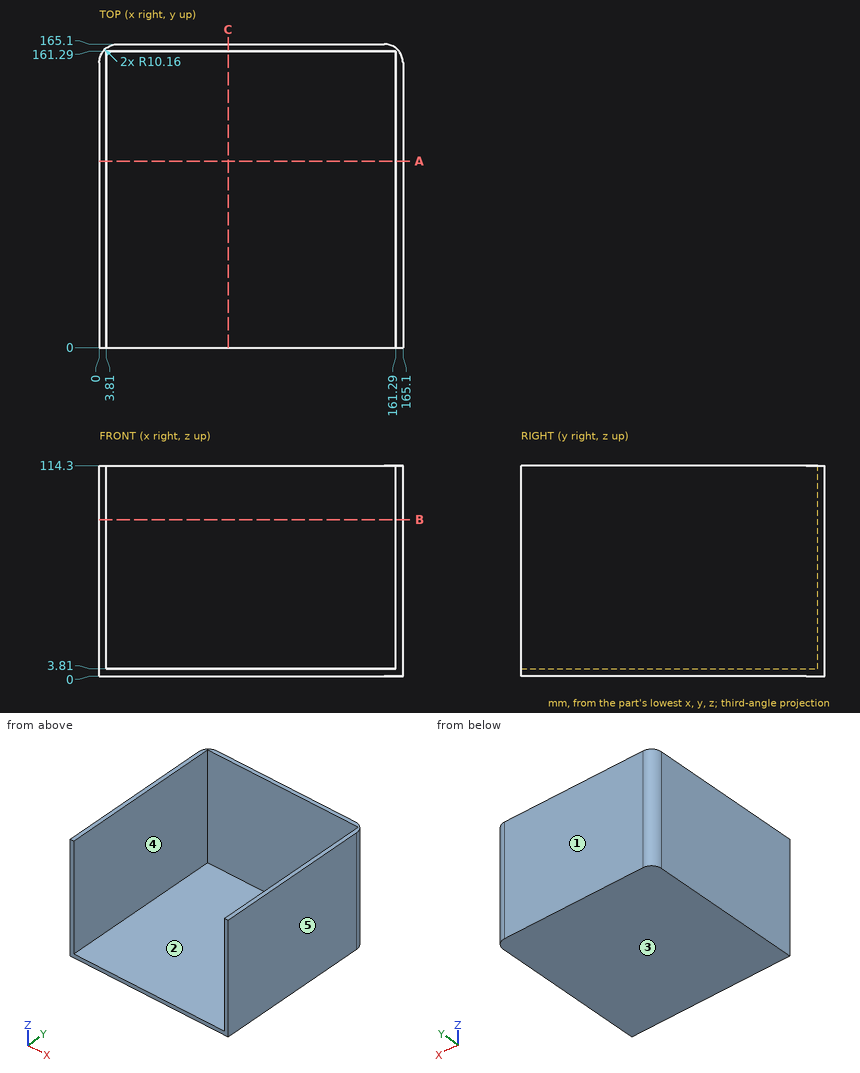
Can you work these out from the drawing? Everything is in mm from the part's minimum corner. A direction names the side the tool comes from. Round coordinates to 2 decimals unless told otherwise and drop trailing zeros. Loops run counter-clockwise (first coordinate to the right, second up) from the corner with the lowest first, then second, coordinate; pieces in that order, holes last. Notation, with made-up numbers: (79.25, 53.5) - (137.25, 53.5) arc R8 ccw to (137.25, 60.5) - close; hole circle Ø8 at (35, 25.25). An arc over 180 degrees is marked (long way). Answer in a Markdown table with one row per item. Add a question column.
Q1. For pin 1 Ø2 at (x, y) = (85.5, 140) entering from +Z, with a flat end and sliding along its axis, tell me the tip position at first contact or that it passes through.
Q2. Which directions (+Z, -Z, +X, -X, +Y, -Y) give clear straight access to the entire face, cutting with the end or side of a thin tool? Please do the marked faces 1 and 2.
Q3. I want a section at C-C on x = 70. List the corners of the cut face in (y, z) for me.
Q4. I want a section at A-A on y = 101.5. List the corners of the cut face in (x, z) for me, and give its area (3 significant figures).
Q5. I want a section at B-B on z = 85. List the corners of the cut face in (x, y) for me.
Q6. We'd pull the mould along X, two halves only. Please class the marked faces 3, 4 and 5: pulls with the +X half, pulls with the -X half, needs draft (parallel to the pull), parting line crosses it, or undercut.
Q7. I need wall thicknesses on L1, parallel to X at y = 40.5, z = 33.5; L2, parallel to Y at x = 104.5, z = 67.5; L3, parallel to Z at x = 141, y = 25. Which ranges of each line are inside material? Lowest first, please.
A:
| question | item | result |
|---|---|---|
| 1 | pin 1 | z = 3.81 |
| 2 | face 1 | +Z, -Z, +X, -X, +Y |
| 2 | face 2 | +Z, -Y |
| 3 | outline | (0, 0) - (165.1, 0) - (165.1, 114.3) - (161.29, 114.3) - (161.29, 3.81) - (0, 3.81) - close |
| 4 | outline | (0, 0) - (165.1, 0) - (165.1, 114.3) - (161.29, 114.3) - (161.29, 3.81) - (3.81, 3.81) - (3.81, 114.3) - (0, 114.3) - close |
| 4 | area | 1,470 mm^2 |
| 5 | outline | (0, 0) - (3.81, 0) - (3.81, 161.29) - (161.29, 161.29) - (161.29, 0) - (165.1, 0) - (165.1, 154.94) arc R10.16 ccw to (154.94, 165.1) - (10.16, 165.1) arc R10.16 ccw to (0, 154.94) - close |
| 6 | face 3 | needs draft |
| 6 | face 4 | undercut |
| 6 | face 5 | pulls with the +X half |
| 7 | L1 | 0 to 3.81, 161.29 to 165.1 |
| 7 | L2 | 161.29 to 165.1 |
| 7 | L3 | 0 to 3.81 |
